Design review of the part built by this model. Coordinates are the model's own, in mm. Coordinates: 2 decimals unless noted, no trailing zeros. Order: outer loops, then holes, each group sorted by start corner. A loop starts at its lowest first (then second) coordinate and runs counter-clockwise, first axis right, second up. Notation, with made-up numbers: M -25.75,79 L 22.25,79 A31 ccw 22.25,111 Z; hole C 50,-18.5 d4. An arc over 180 degrees is marked long. Answer as a JSON object with one key per item and string values.
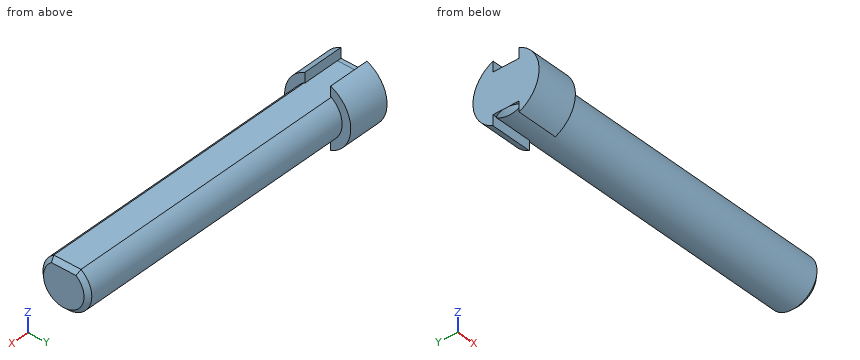
Autodesk Inventor part; units mm, degrees
ref_plane "YZ Plane" through (0, 0, 0) normal (1, 0, 0) x (0, 1, 0)
ref_plane "XZ Plane" through (0, 0, 0) normal (0, 1, 0) x (-1, 0, 0)
ref_plane "XY Plane" through (0, 0, 0) normal (0, 0, 1) x (1, 0, 0)
sketch "Sketch1" plane through (0, 0, 0) normal (1, 0, 0) x (0, 1, 0)
  circle A0 centre (0, 0) radius 2.95
  line L0 (1.6432, 2.45) -> (-1.6432, 2.45)
  dimension "d0" = 5.9
  dimension "d1" = 0.5
extrude "Extrusion1" add sketch "Sketch1" along normal blind 40 contours A0 L0 picked at (0.5577, 0.5097)
chamfer "Chamfer1" distance 0.5 angle 45 4 edges at (0, 0, -2.95) (0, 0, 2.45) (40, 0, -2.95) (40, 0, 2.45)
sketch "Sketch2" plane through (0, 0, 0) normal (-1, 0, 0) x (0, 0, 1)
  circle A0 centre (0, 0) radius 3
  circle A1 centre (0, 0) radius 4
  line L0 (5.565, 1.565) -> (2.435, 1.565)
  line L1 (2.435, 1.565) -> (2.435, -1.565)
  line L2 (2.435, -1.565) -> (5.565, -1.565)
  line L3 (5.565, -1.565) -> (5.565, 1.565)
  line L4 (5.565, 1.565) -> (2.435, -1.565) construction
  line L5 (2.435, 1.565) -> (5.565, -1.565) construction
  line L6 (-2.425, 1.575) -> (-5.575, 1.575)
  line L7 (-5.575, 1.575) -> (-5.575, -1.575)
  line L8 (-5.575, -1.575) -> (-2.425, -1.575)
  line L9 (-2.425, -1.575) -> (-2.425, 1.575)
  line L10 (-2.425, 1.575) -> (-5.575, -1.575) construction
  line L11 (-5.575, 1.575) -> (-2.425, -1.575) construction
  point P0 (4, 0)
  point P1 (-4, 0)
  point P2 (-3.6769, 1.575)
  point P3 (-3.6769, -1.575)
  point P4 (3.6811, -1.565)
  point P5 (3.6811, 1.565)
  dimension "d7" = 3.13
  dimension "d8" = 3.13
  dimension "d9" = 3.15
  dimension "d10" = 3.15
extrude "Extrusion2" add sketch "Sketch2" against normal blind 5 contours L0 L1 L2 A0 L8 L9 L6 | A0 L6 A1 L0 | L2 A1 L8 A0
properties part number "Ø6x40Shaft"
1) To check wall thickness, follow L1, parallel to X at y = -3.25, z = 0.75; L2, parallel to Z at x = 25.5, y = -2.5; L3, parallel to Y at x = 3.5, z = -3.5 (1 decimal). State the ranges of each line that lie inside material, in increasing order.
Taken from the geometry:
{"L1": "x = 0 to 5", "L2": "z = -1.57 to 1.57", "L3": "y = -1.9 to -1.6, 1.6 to 1.9"}
2) Add section B-B (z = 0). State the section outline as (x, y) points, and give its area (3 significant figures).
Taken from the geometry:
{"outline": "M 0,-4 L 5,-4 L 5,-2.95 L 39.5,-2.95 L 40,-2.45 L 40,2.45 L 39.5,2.95 L 5,2.95 L 5,4 L 0,4 Z", "area": "246 mm2"}
3) Add section C-C (x = 18.5). State the section outline as (y, z) points.
Taken from the geometry:
{"outline": "M -1.64,2.45 A2.95 ccw long 1.64,2.45 Z"}
4) Insertion check: pin 1 Ø2.5 at (y, z) = (3, 0) entering from +X; pin 2 Ø2.5 at (x, y) = (21.5, -0.5) entering from +Z; pin 3 Ø0.6 at (x, z) = (3, 3) entering from +Y; pin 4 Ø1.4 at (x, z) = (2.5, 3) entering from -Y. Each pin has a flat end and moves straight along its axis. Give the tip position at first contact, or say it passes through.
Taken from the geometry:
{"pin 1": "stops at x = 40", "pin 2": "stops at z = 2.45", "pin 3": "stops at y = 2.95", "pin 4": "stops at y = -3.27"}
